Work out the finished part from the listing and answer in its coordinate system (mm). A direction names the side the tool comes from. Round coordinates to 2 decimals unless told otherwise and drop trailing zeros. Write each loop counter-clockwise with the first axis right and the second up, starting at its lowest first coordinate (ties: lowest second). Pieces come first, ordered by that corner, then holes. Notation, with made-up numbers: (58.5, -10) -> (102.5, -10) arc R21 ccw to (102.5, 11) -> close; hole circle Ø2 at (-10.5, -35). An arc over 180 degrees is marked (long way). One line per item, written item: value.
```python
from build123d import *

# Parameters (mm, degrees)
F0_W     = 210
F0_H     = 160
F1_DEPTH = 180
F2_T     = -4
F3_W     = 210
F3_H     = 160
F3_W_2   = 191.999994
F3_H_2   = 141.999994
F4_DEPTH = 5


with BuildPart() as f1:
    # F0 (on Top) → F1 (new body)
    with BuildSketch(Plane.XY):
        Rectangle(F0_W, F0_H)
    extrude(amount=F1_DEPTH)

    # F2
    f2_openings = [f1.faces().sort_by_distance(p)[0] for p in [
        (0, 0, 180),
        (0, 0, 0),
    ]]
    offset(amount=F2_T, openings=f2_openings)

    # F3 (on face) → F4 (join)
    with BuildSketch(Plane.XY.offset(180)):
        Rectangle(F3_W, F3_H)
        Rectangle(F3_W_2, F3_H_2, mode=Mode.SUBTRACT)
    extrude(amount=-F4_DEPTH)


solid = f1.part
```
(1) For a pull along Y with two mould halves and no side action, classify faces 1 (the face through (105, -1, 89)), 2 (the face through (-1, -80, 89)), 3 (the face through (-96, -1, 178)), 4 (the face through (-8, -73, 175)) as pulls with the +Y half, pulls with the -Y half, needs draft (parallel to the pull), parting line crosses it, or undercut.
Reported:
face 1: needs draft
face 2: pulls with the -Y half
face 3: undercut
face 4: undercut
(2) Find section C-C on y = -67.5. Give the vertices of the cut face in (x, z), plus the area to 3 significant figures.
Reported:
outline: (-105, 0) -> (-101, 0) -> (-101, 175) -> (-96, 175) -> (-96, 180) -> (-105, 180) -> close; (96, 175) -> (101, 175) -> (101, 0) -> (105, 0) -> (105, 180) -> (96, 180) -> close
area: 1,490 mm2
(3) Consider probe 1 along X at (y, z) = (47, 103); probe 2 along Y at (x, z) = (-71, 9). Determine where each line is inside the solid, lowest interval first.
Reported:
probe 1: x = -105 to -101, 101 to 105
probe 2: y = -80 to -76, 76 to 80
(4) Find section A-A on x = -32.5. Give the vertices of the cut face in (y, z).
Reported:
outline: (-80, 0) -> (-76, 0) -> (-76, 175) -> (-71, 175) -> (-71, 180) -> (-80, 180) -> close; (71, 175) -> (76, 175) -> (76, 0) -> (80, 0) -> (80, 180) -> (71, 180) -> close
(5) Find section B-B on z = 166. Give the vertices of the cut face in (x, y), plus the area to 3 significant figures.
Reported:
outline: (-105, -80) -> (105, -80) -> (105, 80) -> (-105, 80) -> close; hole (-101, -76) -> (101, -76) -> (101, 76) -> (-101, 76) -> close
area: 2,900 mm2
(6) A tool of negligible diameter and unlimited length cuts with its end or side. For faces 5 (the face through (-0.5, 71.5, 180)), 6 (the face through (96, -1, 178)), 7 (the face through (101, -1, 86)), from which of +Z, -Z, +X, -X, +Y, -Y can it reach the whole face along a straight path? Write none if from no direction.
Reported:
face 5: +Z, +X, -X, +Y, -Y
face 6: +Z, -Z
face 7: -Z
